from build123d import *

# Parameters (mm, degrees)
SKETCH_R        = 40
PAD_DEPTH       = 26
SKETCH001_R     = 40
SKETCH001_R_2   = 37.5
POCKET_DEPTH    = 26
SKETCH002_W     = 18.3
SKETCH002_H     = 2
PAD001_DEPTH    = 2
SKETCH003_W     = 18.3
SKETCH003_H     = 2
PAD002_DEPTH    = 2
CHAMFER_SIZE    = 2
CHAMFER001_SIZE = 0.9


with BuildPart() as part:
    # Sketch → Pad (new body)
    with BuildSketch(Plane.XY):
        Circle(SKETCH_R)
        with BuildLine():
            ThreePointArc((26.462757, 9.15), (0, 28), (-26.462757, 9.15))
            Line((-26.362757, 9.15), (-26.462757, 9.15))
            Line((-26.362757, -9.15), (-26.362757, 9.15))
            Line((-26.462757, -9.15), (-26.362757, -9.15))
            ThreePointArc((-26.462757, -9.15), (0, -28), (26.462757, -9.15))
            Line((26.462757, -9.15), (26.362757, -9.15))
            Line((26.362757, -9.15), (26.362757, 9.15))
            Line((26.362757, 9.15), (26.462757, 9.15))
        make_face(mode=Mode.SUBTRACT)
    extrude(amount=PAD_DEPTH)

    # Sketch001 → Pocket (cut)
    with BuildSketch(Plane.XY.offset(27)):
        Circle(SKETCH001_R)
        Circle(SKETCH001_R_2, mode=Mode.SUBTRACT)
    extrude(amount=-POCKET_DEPTH, mode=Mode.SUBTRACT)

    # Sketch002 (on Face10 of Pocket) → Pad001 (join)
    with BuildSketch(Plane.YZ.offset(-26.362757)):
        with Locations((0, 25)):
            Rectangle(SKETCH002_W, SKETCH002_H)
    extrude(amount=PAD001_DEPTH)

    # Sketch003 (on Face6 of Pad001) → Pad002 (join)
    with BuildSketch(Plane(origin=(26.362757, 0, 0), x_dir=(0, -1, 0), z_dir=(-1, 0, 0))):
        with Locations((0, 25)):
            Rectangle(SKETCH003_W, SKETCH003_H)
    extrude(amount=PAD002_DEPTH)

    # Chamfer
    chamfer_edges = [part.edges().sort_by_distance(p)[0] for p in [
        (-37.5, 0, 26),
    ]]
    chamfer(chamfer_edges, length=CHAMFER_SIZE)

    # Chamfer001
    chamfer001_edges = [part.edges().sort_by_distance(p)[0] for p in [
        (-40, 0, 0),
    ]]
    chamfer(chamfer001_edges, length=CHAMFER001_SIZE)


solid = part.part
Part model, mm, in its own coordinate system. A direction names the side the tool comes from. Give positions to 0.01 mm unless a question says otherwise; leave off trailing zeros. Order: outer loops, then holes, each group sorted by start corner. A loop starts at its lowest first (then second) coordinate and runs counter-clockwise, first axis right, second up. Notation, with made-up numbers: (-33, 88) - (-22, 88) arc R25 cw to (-22, 107) - close; hole circle Ø6 at (70.25, 34). An arc over 180 degrees is marked (long way). Use a Markdown table: item, result.
1) Saw through at B-B on y = 0. List the corners of the cut face in (x, z).
Checked values:
| item | result |
|---|---|
| outline | (-40, 0.9) - (-39.1, 0) - (-26.36, 0) - (-26.36, 24) - (-24.36, 24) - (-24.36, 26) - (-35.5, 26) - (-37.5, 24) - (-37.5, 1) - (-40, 1) - close; (24.36, 24) - (26.36, 24) - (26.36, 0) - (39.1, 0) - (40, 0.9) - (40, 1) - (37.5, 1) - (37.5, 24) - (35.5, 26) - (24.36, 26) - close |
2) Probe L1, parallel to X at y = 1, z = 3; L2, parallel to Y at x = -9.5, z = 11.25; L3, parallel to Y at x = -14.5, z = 8.5. List the from-to ranges inside material, lowest first. Write a range as from..to.
Checked values:
| item | result |
|---|---|
| L1 | -37.49..-26.36, 26.36..37.49 |
| L2 | -36.28..-26.34, 26.34..36.28 |
| L3 | -34.58..-23.95, 23.95..34.58 |
3) Two-plate mould, pull along X, no slides. Class faces 1 (the flat face through (12, 36, 1)), 2 (the flat face through (-26.363, 0, 12)), 3 (the flat face through (24.363, 0, 25)), 4 (the cylindrical face through (-4.88, 37.18, 12.66)): +X half, -X half, draft (parallel to the pull), parting line (faces both ways), or undercut.
Checked values:
| item | result |
|---|---|
| face 1 | draft |
| face 2 | undercut |
| face 3 | undercut |
| face 4 | parting line |
4) Saw through at A-A on x = 0. List the corners of the cut face in (y, z), plus the area to 3 significant figures.
Checked values:
| item | result |
|---|---|
| outline | (-40, 0.9) - (-39.1, 0) - (-28, 0) - (-28, 26) - (-35.5, 26) - (-37.5, 24) - (-37.5, 1) - (-40, 1) - close; (28, 0) - (39.1, 0) - (40, 0.9) - (40, 1) - (37.5, 1) - (37.5, 24) - (35.5, 26) - (28, 26) - close |
| area | 494 mm² |
5) Flat gauge pins, fed straight in: P1, Ø2, axis at y = 10.5, z = 20.5, coming from the +X side; P2, Ø0.6, axis at x = -25, y = 2, coming from the -Z side; P3, Ø2, axis at x = 10.5, z = 15.5, coming from the +Y side; P4, Ø14.5, axis at y = 1.5, z = 8, coming from the -X side. Where does each tip first touch, or does it go through?
Checked values:
| item | result |
|---|---|
| P1 | x = 36.28 |
| P2 | z = 24 |
| P3 | y = 36.28 |
| P4 | x = -40 |
6) 3-axis set-ups, long thin cutter, end or side, ignore diameter. For faces 5 (the flat face through (-24.363, 0, 25)), 6 (the flat face through (25, 0, 24)), 7 (the flat face through (-26, 0, 26)): which of +Z, -Z, +X, -X, +Y, -Y reach the whole face in a straight line?
Checked values:
| item | result |
|---|---|
| face 5 | +Z, -Z |
| face 6 | -Z |
| face 7 | +Z, +X, -X, +Y, -Y |
7) Saw through at C-C on z = 5.25. List the corners of the cut face in (x, y), plus the area to 3 significant figures.
Checked values:
| item | result |
|---|---|
| outline | circle Ø75 at (0, 0); hole (-26.46, -9.15) arc R28 ccw to (26.46, -9.15) - (26.36, -9.15) - (26.36, 9.15) - (26.46, 9.15) arc R28 ccw to (-26.46, 9.15) - (-26.36, 9.15) - (-26.36, -9.15) - close |
| area | 2,000 mm² |
